Verification items for the finished model (mm, model axes). Face numbers are marked on the shaded views. A direction names the side the tool comes from. Round coordinates to 2 decimals unless told otherwise and drop trailing zeros. Write each loop counter-clockwise with the first axis right and the second up, starting at its lowest first coordinate (ties: lowest second). Pieces come first, ordered by that corner, then holes. Notation, with made-up numbers: M 29,-15.5 L 61,-15.5 A15 cw 61,7.5 Z; hole C 8,14 d5. An arc over 180 degrees is marked long. Answer in a Markdown table with one row per item. Add a question column.
1. Sectioned sample at B-B on z = -2. Record the cut outline in (x, y).
2. Set-up check for the marked faces 1 and 2: record each of +Z, -Z, +X, -X, +Y, -Y from which the full face is reachable in a straight line by a thin tool's end or side.
3. Sectioned sample at C-C on z = 1.5. Record the cut outline in (x, y), plus the area to 3 significant figures.
4. Material ranges on probe 1 along Z at (x, y) = (5.25, -2.5); probe 2 along X at (y, z) = (1.75, -4); probe 3 along Z at (x, y) = (-3.25, 0.75), recorded low to high.
5. Sectioned sample at D-D on z = 0.5. Record the cut outline in (x, y), plus the area to 3 significant figures.
6. Go/stop test with flat-tipped pins: pin 1 Ø1 at (x, z) = (-4.5, 0) entering from +Y; pin 2 Ø2 at (x, y) = (-2.5, 4) entering from -Z. Record where each tip stops, or that it passes through.
7. Sectioned sample at A-A on x = 0. Record the cut outline in (y, z), plus the area to 3 significant figures.
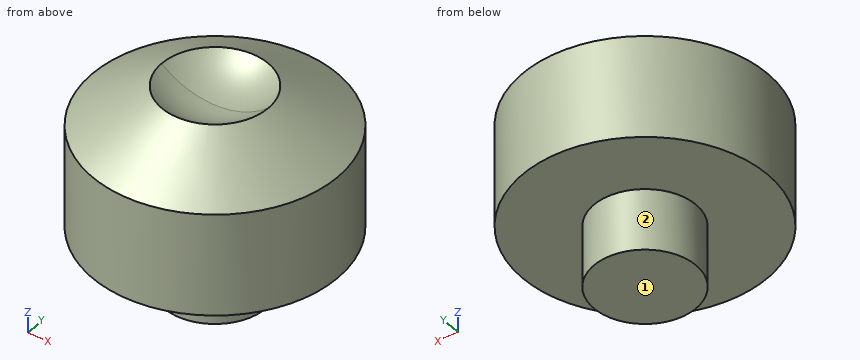
```python
from build123d import *
from build123d.topology import SkipClean

# Parameters (mm, degrees)
SKETCH2_R           = 6
BOSS_EXTRUDE1_DEPTH = 2
CHAMFER1_SIZE       = 2
CHAMFER1_SIZE_2     = 3.464101615
SKETCH4_R           = 6
BOSS_EXTRUDE2_DEPTH = 5
SKETCH6_R           = 2.5
BOSS_EXTRUDE3_DEPTH = 3


with BuildPart() as part:
    # Sketch2 → Boss-Extrude1 (new body)
    with BuildSketch(Plane.XY):
        Circle(SKETCH2_R)
    extrude(amount=BOSS_EXTRUDE1_DEPTH)

    # Sketch3 one side → Cut-Revolve1 (revolve, cut)
    with SkipClean():  # the faces are left unmerged after this step: merging them gives an invalid solid
        with BuildSketch(Plane(origin=(0, 0, 0), x_dir=(0, 0, -1), z_dir=(1, 0, 0))):
            with BuildLine():
                ThreePointArc((-5, -4), (-2.171572875, -2.828427125), (-1, 0))
                ThreePointArc((-1, 0), (-2.171572875, 2.828427125), (-5, 4))
                Line((-5, 4), (-5, -4))
            make_face()
        revolve(axis=Axis((0, 4, 5), (0, -1, 0)), mode=Mode.SUBTRACT)

    # Chamfer1
    # the kernel refuses this chamfer: 3.464101615, 2 mm, written as the material it takes off along each edge
    with BuildSketch(Plane(origin=(0, 0, 2), x_dir=(1, 0, 0), z_dir=(0, -1, 0))) as chamfer1_piece_1:
        Polygon((6, -CHAMFER1_SIZE), (6 - CHAMFER1_SIZE_2, 0), (6, 0), align=None)
    revolve(axis=Axis((0, 0, 2), (0, 0, 1)), mode=Mode.SUBTRACT)

    # Sketch4 → Boss-Extrude2 (add)
    with BuildSketch(Plane(origin=(0, 0, 0), x_dir=(-1, 0, 0), z_dir=(0, 0, -1))):
        Circle(SKETCH4_R)
    extrude(amount=BOSS_EXTRUDE2_DEPTH)

    # Sketch6 → Boss-Extrude3 (add)
    with BuildSketch(Plane(origin=(0, 0, -5), x_dir=(-1, 0, 0), z_dir=(0, 0, -1))):
        Circle(SKETCH6_R)
    extrude(amount=BOSS_EXTRUDE3_DEPTH)


solid = part.part
```
Geometry check:
| question | item | result |
|---|---|---|
| 1 | outline | C 0,0 d12 |
| 2 | face 1 | -Z, +X, -X, +Y, -Y |
| 2 | face 2 | -Z |
| 3 | outline | C 0,0 d6.8; hole C 0,0 d3.87 |
| 3 | area | 24.6 mm2 |
| 4 | probe 1 | z = -5 to 0.11 |
| 4 | probe 2 | x = -5.74 to 5.74 |
| 4 | probe 3 | z = -5 to 1.54 |
| 5 | outline | C 0,0 d10.27 |
| 5 | area | 82.8 mm2 |
| 6 | pin 1 | stops at y = 4.47 |
| 6 | pin 2 | stops at z = -5 |
| 7 | outline | M -6,-5 L -2.5,-5 L -2.5,-8 L 2.5,-8 L 2.5,-5 L 6,-5 L 6,0 L 2.6,1.96 A4 cw -2.6,1.96 L -6,0 Z |
| 7 | area | 88.4 mm2 |
